The model under review builds one solid part; all positions refer to its coordinate system, in mm. Face numbers are marked on the shaded views. A direction names the side the tool comes from. Round coordinates to 2 decimals unless told otherwise and drop trailing zeros. Order: outer loops, then holes, each group sorted by start corner. A loop starts at its lowest first (then second) coordinate and runs counter-clockwise, first axis right, second up.
1) Machinability: for the marked faces 1, 2 and 3, which of the approach directions +Z, -Z, +X, -X, +Y, -Y give a long, thin tool a straight path to every point of the face, cutting with its end or side? Answer none if there is none.
2) Consider section B-B (z = 8). Give the boundary of the cut face in (x, y), then the cut area to 3 significant figures.
3) Clearance check with flat-ended pins moving along their axes: P1, Ø5, axis at x = 63.5, y = 11.5, coming from the -Z side; P2, Ø8, axis at y = -0.5, z = 2.5, coming from the +X side; P3, Ø12, axis at x = 117.5, z = -42, coming from the +Y side; P4, Ø9, axis at x = 69.596, y = -12.7, coming from the -Z side. State where each tip first meets the part, or that it passes through.
4) Consider section C-C (x = 35.5). Give the boundary of the cut face in (y, z), then the cut area to 3 significant figures.
5) Consider section A-A (y = 12.7). Give the boundary of the cut face in (x, z).
6) Mouldability with a two-part tool opening along Y and no side actions: class the marked faces 4, 5 and 6 as pulls with the +Y half, pulls with the -Y half, needs draft (parallel to the pull), parting line crosses it, or undercut.
7) Consider section D-D (z = -25). Give the boundary of the cut face in (x, y), then the cut area to 3 significant figures.
8) To check wall thickness, follow L1, parallel to Z at x = 57, y = -21; L2, parallel to X at y = 12, z = 9; L3, parallel to Y at x = 70.5, z = 8.5. State the ranges of each line that lie inside material, in increasing order.
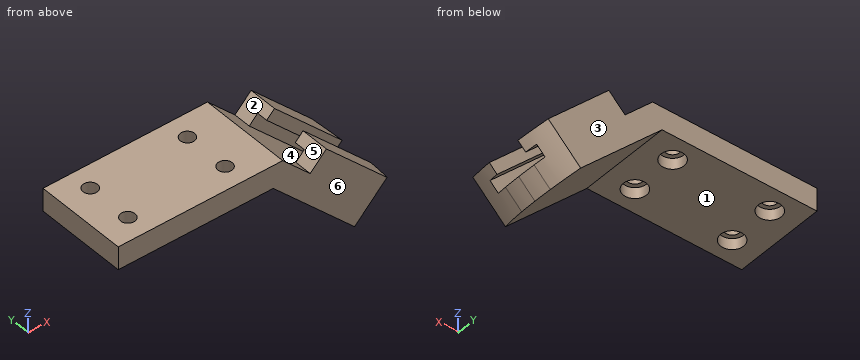
from build123d import *

# Parameters (mm, degrees)
F1_DEPTH       = 25.4
F4_D           = 7.9248
F4_CBORE_D     = 12.7
F4_CBORE_DEPTH = 6.096
F6_DEPTH       = 139.7917874995
F8_DEPTH       = 121.1595313784


with BuildPart() as f1:
    # F0 (on Front) → F1 (new body, symmetric)
    with BuildSketch(Plane.XZ):
        Polygon((0, 12.7), (0, 0), (85.852, 0), (135.4230137883, -49.5710137883), (153.3835260304, -31.6105015462), (115.3072400771, 6.4657844072), (106.326983956, -2.5144717139), (91.1125122421, 12.7), align=None)
    extrude(amount=F1_DEPTH, both=True)

    # F4 (through all)
    with Locations(Plane(origin=(0, 0, 0), x_dir=(1, 0, 0), z_dir=(0, 0, -1))):
        with Locations((15.748, 12.7), (15.748, -12.7), (69.596, 12.7), (69.596, -12.7)):
            CounterBoreHole(F4_D / 2, F4_CBORE_D / 2, F4_CBORE_DEPTH)

    # F5 (on face) → F6 (cut, through all)
    with BuildSketch(Plane(origin=(92.4970137883, 0, -92.4970137883), x_dir=(0, 1, 0), z_dir=(0.7071067812, 0, -0.7071067812))):
        Polygon((9.652, 86.1065313784), (-9.652, 86.1065313784), (-9.652, 80.0105313784), (-15.748, 80.0105313784), (-15.748, 73.4065313784), (15.748, 73.4065313784), (15.748, 80.0105313784), (9.652, 80.0105313784), align=None)
    extrude(amount=-F6_DEPTH, mode=Mode.SUBTRACT)

    # F7 (on face) → F8 (cut, through all)
    with BuildSketch(Plane(origin=(60.8865122421, 0, 60.8865122421), x_dir=(0.7071067812, 0, -0.7071067812), z_dir=(0.7071067812, 0, 0.7071067812))):
        with BuildLine():
            ThreePointArc((129.9384315595, -9.652), (127.8044235189, -17.7400424907), (124.4435497331, -25.4))
            Line((124.4435497331, -25.4), (130.8105313784, -25.4))
            Line((130.8105313784, -25.4), (130.8105313784, -15.748))
            Line((130.8105313784, -15.748), (130.8105313784, -9.652))
            Line((130.8105313784, -9.652), (129.9384315595, -9.652))
        make_face()
        with BuildLine():
            Line((129.9384315595, 9.652), (130.8105313784, 9.652))
            Line((130.8105313784, 9.652), (130.8105313784, 15.748))
            Line((130.8105313784, 15.748), (130.8105313784, 25.4))
            Line((130.8105313784, 25.4), (124.4435497331, 25.4))
            ThreePointArc((124.4435497331, 25.4), (127.8044235189, 17.7400424907), (129.9384315595, 9.652))
        make_face()
        with BuildLine():
            ThreePointArc((130.8105313784, 0), (130.5920632473, -4.8456594519), (129.9384315595, -9.652))
            Line((129.9384315595, -9.652), (130.8105313784, -9.652))
            Line((130.8105313784, -9.652), (130.8105313784, 0))
        make_face()
        with BuildLine():
            ThreePointArc((129.9384315595, 9.652), (130.5920632473, 4.8456594519), (130.8105313784, 0))
            Line((130.8105313784, 0), (130.8105313784, 9.652))
            Line((130.8105313784, 9.652), (129.9384315595, 9.652))
        make_face()
    extrude(amount=-F8_DEPTH, mode=Mode.SUBTRACT)


solid = f1.part
Answer below:
1. face 1: -Z, -X, +Y, -Y
1. face 2: +Z, +Y, -Y
1. face 3: +Z, -Z, +X, -X, +Y
2. outline: (0, -25.4) - (95.81, -25.4) - (95.81, 25.4) - (0, 25.4) - close; hole circle Ø7.92 at (15.75, -12.7); hole circle Ø7.92 at (15.75, 12.7); hole circle Ø7.92 at (69.6, -12.7); hole circle Ø7.92 at (69.6, 12.7)
2. area: 4,670 mm2
3. P1: stops at z = 0
3. P2: stops at x = 105.31
3. P3: passes through
3. P4: stops at z = 6.1
4. outline: (-25.4, 0) - (25.4, 0) - (25.4, 12.7) - (-25.4, 12.7) - close
4. area: 645 mm2
5. outline: (0, 0) - (9.4, 0) - (9.4, 6.1) - (11.79, 6.1) - (11.79, 12.7) - (0, 12.7) - close; (19.71, 6.1) - (22.1, 6.1) - (22.1, 0) - (63.25, 0) - (63.25, 6.1) - (65.63, 6.1) - (65.63, 12.7) - (19.71, 12.7) - close; (73.56, 6.1) - (75.95, 6.1) - (75.95, 0) - (85.85, 0) - (134.35, -48.5) - (143.33, -39.52) - (91.11, 12.7) - (73.56, 12.7) - close; (111, 2.16) - (148, -34.85) - (152.31, -30.54) - (115.31, 6.47) - close
6. face 4: undercut
6. face 5: needs draft
6. face 6: pulls with the -Y half
7. outline: (110.85, -25.4) - (146.77, -25.4) - (146.77, -9.65) - (138.15, -9.65) - (138.15, -15.75) - (128.81, -15.75) - (128.81, 15.75) - (138.15, 15.75) - (138.15, 9.65) - (146.77, 9.65) - (146.77, 25.4) - (110.85, 25.4) - close
7. area: 1,360 mm2
8. L1: z = 0 to 12.7
8. L2: x = 0 to 11.85, 19.65 to 65.7, 73.5 to 94.81
8. L3: y = -25.4 to -16.56, -8.84 to 8.84, 16.56 to 25.4
